Read the model definition and answer for the solid it produces. Units are mm, in the model's axes. Coordinates: 2 decimals unless noted, no trailing zeros. Loops run counter-clockwise (first coordinate to the right, second up) from the corner with the lowest first, then second, coordinate; pieces in that order, holes last. Notation, with made-up numbers: (19, 75.25) - (36, 75.25) arc R36 cw to (36, 109.25) - close; hole circle Ø5 at (64.25, 63.5). An arc over 180 degrees is marked (long way). Use one line per item in the form item = value. Start each with the question number.
1) A cutting plane is placed at B-B (z = 6.5). Give the vertices of the cut face in (x, y), and give its area (3 significant figures).
2) A cutting plane is placed at A-A (x = -51.5). Give the vertices of the cut face in (y, z).
3) Consider line 1 (X direction, y = 1.95, z = -29); line 2 (X direction, y = 1.8, z = -27.5); line 3 (Z direction, x = -44.5, y = 0.2). Determine where each line is inside the solid, lowest interval first.
4) Each of these flat-tipped pins is pushed along its axis until it touches: P1, Ø0.7, axis at x = -14.5, y = 2, coming from the -Z side; P2, Ø0.9, axis at y = 2, z = -30.5, coming from the -X side; P3, Ø0.9, axis at x = -60, y = 1.5, coming from the -Z side. Where does it stop, or does it pass through?
5) A cutting plane is placed at D-D (x = -31). Give the vertices of the cut face in (y, z).
6) A cutting plane is placed at C-C (z = -2.5). Give the vertices of the cut face in (x, y).
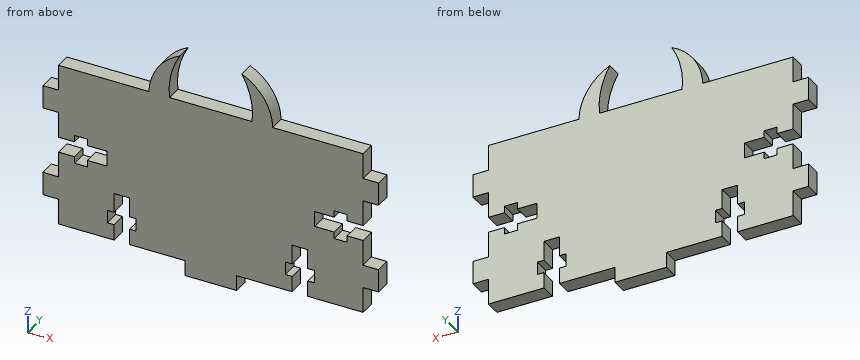
from build123d import *

# Parameters (mm, degrees)
BOSS_EXTRUDE1_DEPTH = 3


with BuildPart() as part:
    # Sketch1 → Boss-Extrude1 (new body)
    with BuildSketch(Plane(origin=(0, 0, 0), x_dir=(1, 0, 0), z_dir=(0, 1, 0))):
        with BuildLine():
            Line((0, 27), (3, 27))
            Line((3, 27), (3, 22.5))
            Line((3, 22.5), (0, 22.5))
            Line((0, 22.5), (0, 17.5))
            Line((0, 17.5), (-3.1, 17.5))
            Line((-3.1, 17.5), (-3.1, 18.8))
            Line((-3.1, 18.8), (-5.6, 18.8))
            Line((-5.6, 18.8), (-5.6, 17.5))
            Line((-5.6, 17.5), (-9.4, 17.5))
            Line((-9.4, 17.5), (-9.4, 14.5))
            Line((-9.4, 14.5), (-5.6, 14.5))
            Line((-5.6, 14.5), (-5.6, 13.2))
            Line((-5.6, 13.2), (-3.1, 13.2))
            Line((-3.1, 13.2), (-3.1, 14.5))
            Line((-3.1, 14.5), (0, 14.5))
            Line((0, 14.5), (0, 9.5))
            Line((0, 9.5), (3, 9.5))
            Line((3, 9.5), (3, 5))
            Line((3, 5), (0, 5))
            Line((0, 5), (0, 0))
            Line((0, 0), (-17.5, 0))
            ThreePointArc((-17.5, 0), (-19.217483451, -5.355011032), (-23.5, -9))
            ThreePointArc((-23.5, -9), (-21.768352481, -4.662588338), (-21.5, 0))
            Line((-21.5, 0), (-37.5, 0))
            ThreePointArc((-37.5, 0), (-37.231647519, -4.662588338), (-35.5, -9))
            ThreePointArc((-35.5, -9), (-39.782516549, -5.355011032), (-41.5, 0))
            Line((-41.5, 0), (-59, 0))
            Line((-59, 0), (-59, 5))
            Line((-59, 5), (-62, 5))
            Line((-62, 5), (-62, 9.5))
            Line((-62, 9.5), (-59, 9.5))
            Line((-59, 9.5), (-59, 14.5))
            Line((-59, 14.5), (-55.9, 14.5))
            Line((-55.9, 14.5), (-55.9, 13.2))
            Line((-55.9, 13.2), (-53.4, 13.2))
            Line((-53.4, 13.2), (-53.4, 14.5))
            Line((-53.4, 14.5), (-49.6, 14.5))
            Line((-49.6, 14.5), (-49.6, 17.5))
            Line((-49.6, 17.5), (-53.4, 17.5))
            Line((-53.4, 17.5), (-53.4, 18.8))
            Line((-53.4, 18.8), (-55.9, 18.8))
            Line((-55.9, 18.8), (-55.9, 17.5))
            Line((-55.9, 17.5), (-59, 17.5))
            Line((-59, 17.5), (-59, 22.5))
            Line((-59, 22.5), (-62, 22.5))
            Line((-62, 22.5), (-62, 27))
            Line((-62, 27), (-59, 27))
            Line((-59, 27), (-59, 32))
            Line((-59, 32), (-48.25, 32))
            Line((-48.25, 32), (-48.25, 28.9))
            Line((-48.25, 28.9), (-49.55, 28.9))
            Line((-49.55, 28.9), (-49.55, 26.4))
            Line((-49.55, 26.4), (-48.25, 26.4))
            Line((-48.25, 26.4), (-48.25, 22.6))
            Line((-48.25, 22.6), (-45.25, 22.6))
            Line((-45.25, 22.6), (-45.25, 26.4))
            Line((-45.25, 26.4), (-43.95, 26.4))
            Line((-43.95, 26.4), (-43.95, 28.9))
            Line((-43.95, 28.9), (-45.25, 28.9))
            Line((-45.25, 28.9), (-45.25, 32))
            Line((-45.25, 32), (-34.5, 32))
            Line((-34.5, 32), (-34.5, 35))
            Line((-34.5, 35), (-24.5, 35))
            Line((-24.5, 35), (-24.5, 32))
            Line((-24.5, 32), (-13.75, 32))
            Line((-13.75, 32), (-13.75, 28.9))
            Line((-13.75, 28.9), (-15.05, 28.9))
            Line((-15.05, 28.9), (-15.05, 26.4))
            Line((-15.05, 26.4), (-13.75, 26.4))
            Line((-13.75, 26.4), (-13.75, 22.6))
            Line((-13.75, 22.6), (-10.75, 22.6))
            Line((-10.75, 22.6), (-10.75, 26.4))
            Line((-10.75, 26.4), (-9.45, 26.4))
            Line((-9.45, 26.4), (-9.45, 28.9))
            Line((-9.45, 28.9), (-10.75, 28.9))
            Line((-10.75, 28.9), (-10.75, 32))
            Line((-10.75, 32), (0, 32))
            Line((0, 32), (0, 27))
        make_face()
    extrude(amount=BOSS_EXTRUDE1_DEPTH)


solid = part.part
Found:
q1.outline = (-38.9, 0) - (-36.69, 0) - (-36.69, 3) - (-38.9, 3) - close; (-22.31, 0) - (-20.1, 0) - (-20.1, 3) - (-22.31, 3) - close
q1.area = 13.2 mm^2
q2.outline = (0, -32) - (3, -32) - (3, -17.5) - (0, -17.5) - close; (0, -14.5) - (3, -14.5) - (3, 0) - (0, 0) - close
q3.line_1 = -59 to -48.25, -45.25 to -13.75, -10.75 to 0
q3.line_2 = -59 to -49.55, -43.95 to -15.05, -9.45 to 0
q3.line_3 = -32 to -28.9, -26.4 to 0
q4.P1 = -32
q4.P2 = -59
q4.P3 = -27
q5.outline = (0, -35) - (3, -35) - (3, 0) - (0, 0) - close
q6.outline = (-59, 0) - (0, 0) - (0, 3) - (-59, 3) - close
